The model under review builds one solid part; all positions refer to its coordinate system, in mm. Coordinates: 2 decimals unless noted, no trailing zeros. Order: outer loops, then holes, each group sorted by start corner. A loop starts at its lowest first (then second) coordinate and runs counter-clockwise, first axis right, second up. Notation, with made-up numbers: M -13,78.5 L 46,78.5 A18 ccw 46,84.5 Z; hole C -34.75,-7.5 d6. An arc over 180 degrees is marked long. Answer as CSV lines item,"result". Start each with the question number.
Q1. Consider section A-A on y = 4.5. State how many separate pieces and enclosed holes the cut face has, and give its area (3 significant figures).
Q2. Wall thickness on L1, parallel to X at y = 2, z = -38.1; L2, parallel to X at y = 3.75, z = -137.16; L3, parallel to Z at x = 435, y = 5.5: over which ranges is each line inside the solid? List them lowest first. Write a range as [from, to].
Q3. For P1, Ø6.5, axis at x = 303.67, z = -863.73, coming from the -Y side; P2, Ø2, axis at y = 0.5, z = -798, coming from the -X side, all flat-tipped, find the tip position at first contact; note any pin that passes through.
Q4. Consider section C-C on z = -116.5. Write out the cut boundary in (x, y).
Q5. Consider section B-B on x = 360.5. Write out the cut boundary in (y, z), and give its area (3 significant figures).
from build123d import *

# Parameters (mm, degrees)
SKETCH4_R           = 5.3578125
BOSS_EXTRUDE2_DEPTH = 6.35


with BuildPart() as part:
    # Sketch4 → Boss-Extrude2 (new body)
    with BuildSketch(Plane(origin=(0, 0, 0), x_dir=(1, 0, 0), z_dir=(0, 1, 0))):
        Polygon((234.979236566, 1078.971634327), (-356.170330123, 0), (682.689669877, 0), (429.674039163, 609.761730508), (381.000338514, 727.064206463), align=None)
        with Locations((-178.370330123, 38.1)):
            Circle(SKETCH4_R, mode=Mode.SUBTRACT)
        with Locations((-259.300975608, 137.16)):
            Circle(SKETCH4_R, mode=Mode.SUBTRACT)
        with Locations((-93.289784566, 440.165155055)):
            Circle(SKETCH4_R, mode=Mode.SUBTRACT)
        with Locations((504.889669877, 38.1)):
            Circle(SKETCH4_R, mode=Mode.SUBTRACT)
        with Locations((489.29326545, 416.375307605)):
            Circle(SKETCH4_R, mode=Mode.SUBTRACT)
        with Locations((61.094542054, 721.948850069)):
            Circle(SKETCH4_R, mode=Mode.SUBTRACT)
        with Locations((303.667495105, 863.729056592)):
            Circle(SKETCH4_R, mode=Mode.SUBTRACT)
        with Locations((201.97392089, 979.083189991)):
            Circle(SKETCH4_R, mode=Mode.SUBTRACT)
        Polygon((429.674039163, 609.761730508), (381.000338514, 727.064206463), (398.595709907, 734.36526156), (447.269410556, 617.062785606), align=None)
    extrude(amount=BOSS_EXTRUDE2_DEPTH)


solid = part.part
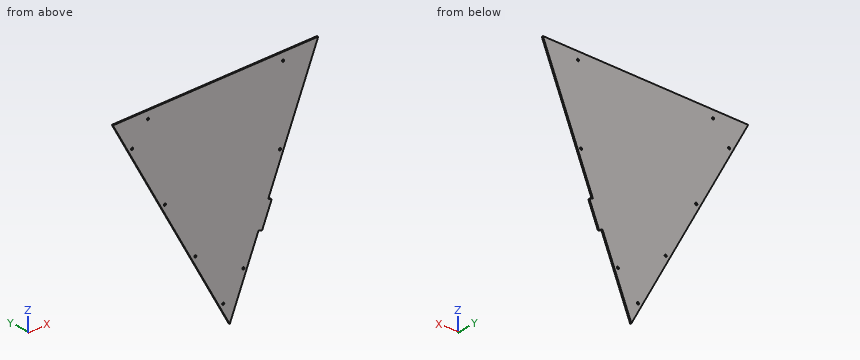
Evaluation:
1,separate pieces,"1"
1,enclosed holes,"8"
1,area,"562,000 mm²"
2,L1,"x = [-335.3, -183.73], [-173.01, 499.53], [510.25, 666.88]"
2,L2,"x = [-281.02, -264.66], [-253.94, 625.78]"
2,L3,"z = [-646.63, -611.97], [-596.93, 0]"
3,P1,"passes through"
3,P2,"stops at x = 80.49"
4,outline,"M -292.34,0 L 634.35,0 L 634.35,6.35 L -292.34,6.35 Z"
5,outline,"M 0,-776.47 L 6.35,-776.47 L 6.35,0 L 0,0 Z"
5,area,"4,930 mm²"
